Input: part model. Units: mm. Frame: model coordinates. A direction names the side the tool comes from. Coordinates: 2 decimals unless noted, no trailing zeros. Loops run counter-clockwise (first coordinate to the right, second up) from the corner with the lowest first, then second, coordinate; pieces in that order, holes last. Notation, with made-up numbers: (2.5, 9) - (41.5, 9) arc R15 ccw to (41.5, 18) - close; hole circle Ø2 at (70, -11.75). An arc over 180 degrees is marked (long way). Use one line per item in the form item = value.
from build123d import *

# Parameters (mm, degrees)
F0_W           = 12.7
F0_H           = 80
F2_W           = 8
F2_H           = 52
F3_DEPTH       = 12.701
F3_DEPTH_BACK  = 12.701
F4_R           = 4
F5_DEPTH       = 5
F6_R           = 2
F7_DEPTH       = 10
F8_R           = 4
F9_R           = 1.55
F10_DEPTH      = 12.7010001
F10_DEPTH_BACK = 12.7010001


with BuildPart() as f1:
    # F0 (on Front) → F1 (revolve)
    with BuildSketch(Plane.XZ):
        with Locations((-6.35, 30)):
            Rectangle(F0_W, F0_H)
    revolve(axis=Axis((0, 0, 30), (0, 0, -1)))

    # F2 (on Right) → F3 (cut, two sides)
    with BuildSketch(Plane.YZ) as f3_sk:
        with Locations((0, 16)):
            Rectangle(F2_W, F2_H)
    extrude(amount=-F3_DEPTH, mode=Mode.SUBTRACT)
    extrude(f3_sk.sketch, amount=F3_DEPTH_BACK, mode=Mode.SUBTRACT)

    # F4 (on Front) → F5 (join, symmetric)
    with BuildSketch(Plane.XZ):
        Circle(F4_R)
    extrude(amount=F5_DEPTH, both=True)

    # F6 (on face) → F7 (cut)
    with BuildSketch(Plane.XY.offset(70)):
        with Locations((-6, 0)):
            Circle(F6_R)
        with Locations((6, 0)):
            Circle(F6_R)
    extrude(amount=-F7_DEPTH, mode=Mode.SUBTRACT)

    # F8
    f8_edges = [f1.edges().sort_by_distance(p)[0] for p in [
        (-12.537366, 2.025944, 42),
        (12.7, 0, 42),
        (-12.537366, -2.025944, 42),
        (0, -12.7, -10),
        (0, 12.7, -10),
    ]]
    fillet(f8_edges, radius=F8_R)

    # F9 (on Front) → F10 (cut, two sides)
    with BuildSketch(Plane.XZ) as f10_sk:
        with Locations((0, 55)):
            Circle(F9_R)
    extrude(amount=F10_DEPTH, mode=Mode.SUBTRACT)
    extrude(f10_sk.sketch, amount=-F10_DEPTH_BACK, mode=Mode.SUBTRACT)


solid = f1.part
Q1. First-contact query: P1, Ø5, axis at y = 2.5, z = 21, coming from the +X side; P2, Ø8, axis at y = -7.5, z = 1, coming from the -X side; P3, Ø6.5, axis at x = -6, y = 0, coming from the +Z side; P4, Ø6, axis at x = 9.5, z = 3.5, coming from the +Y side. Flat tips, straight axial feed; report the tip coordinate or a pass-through.
Check values:
P1 = 12.05
P2 = -12.05
P3 = 70
P4 = 10.91
Q2. Cut plane C-C, the plane z = 29. Return loops of the section in (x, y), then the cut area to 3 significant figures.
Check values:
outline = (-12.05, -4) arc R12.7 ccw to (12.05, -4) - close; (-12.05, 4) - (12.05, 4) arc R12.7 ccw to start
area = 307 mm²
Q3. Pull-direction query (Z, two-part tool) for faces 4 (the flat face through (-6, 0, 60)), 5 (the cylindrical face through (4.4, -1.2, 65.1)), 6 (the cylindrical face through (-0.867, -0.056, -3.905)); classes: pulls with the +Z half, pulls with the -Z half, needs draft (parallel to the pull), parting line crosses it, or undercut.
Check values:
face_4 = pulls with the +Z half
face_5 = needs draft
face_6 = undercut
Q4. Cut plane A-A, the plane y = 0. Return loops of the section in (x, z), then the cut area to 3 significant figures.
Check values:
outline = (-12.7, 46) arc R4 ccw to (-8.7, 42) - (8.7, 42) arc R4 ccw to (12.7, 46) - (12.7, 70) - (8, 70) - (8, 60) - (4, 60) - (4, 70) - (-4, 70) - (-4, 60) - (-8, 60) - (-8, 70) - (-12.7, 70) - close; circle Ø8 at (0, 0); hole circle Ø3.1 at (0, 55)
area = 667 mm²
Q5. Ray query, line 1 along Z through (x, y) = (0, -6); line 2 along Z through (x, y) = (-1.25, -2.75); line 3 along X through (y, z) = (4, 55). Return the intervals inside material, ascending. Write a range as [from, to].
Check values:
line_1 = [-10, 53.45], [56.55, 70]
line_2 = [-3.8, 3.8], [42, 54.08], [55.92, 70]
line_3 = [-12.05, -1.55], [1.55, 12.05]
Q6. Cut plane B-B, the plane x = 0. Return loops of the section in (y, z), then the cut area to 3 significant figures.
Check values:
outline = (-12.7, -6) arc R4 ccw to (-8.7, -10) - (-4, -10) - (-4, -4) - (4, -4) - (4, -10) - (8.7, -10) arc R4 ccw to (12.7, -6) - (12.7, 53.45) - (-12.7, 53.45) - close; (-12.7, 56.55) - (12.7, 56.55) - (12.7, 70) - (-12.7, 70) - close; hole (-4, 4) - (4, 4) - (4, 42) - (-4, 42) - close
area = 1,590 mm²
Q7. Cut plane D-D, the plane z = 0. Return loops of the section in (x, y).
Check values:
outline = (-12.05, -4) arc R12.7 ccw to (12.05, -4) - (4, -4) - (4, 4) - (12.05, 4) arc R12.7 ccw to (-12.05, 4) - (-4, 4) - (-4, -4) - close
Q8. Set-up query: faces 1 (the flat face through (0, 0, 42)), 2 (the cylindrical face through (-5.86, -11.267, 32.532)), 3 (the flat face through (6, 0, 60)). Return all of +Z, -Z, +X, -X, +Y, -Y with unobstructed straight access to the full face (end or side cutting, diameter ignored); none if empty.
Check values:
face_1 = +X, -X
face_2 = +Z, -Z
face_3 = +Z
